Source: CAD feature listing. Evaluate the final solid. Frame: model axes, mm. A direction names the side the tool comes from. Round coordinates to 2 decimals unless told otherwise and drop trailing zeros. Loops run counter-clockwise (first coordinate to the right, second up) from the corner with the lowest first, then second, coordinate; pieces in that order, holes last. Notation, with made-up numbers: (75.25, -38.5) - (99.25, -38.5) arc R8 cw to (99.25, -34.5) - close; hole circle Ø6 at (33, 83.25). An arc over 180 degrees is marked (long way). One line per question, with ' | ' between items.
from build123d import *

# Parameters (mm, degrees)
PAD_DEPTH       = 50
FILLET_R        = 1.5
FILLET001_R     = 1.5
FILLET002_R     = 1.5
FILLET003_R     = 1.5
SKETCH001_R     = 2.1
POCKET_DEPTH    = 50.001
SKETCH002_R     = 2.1
POCKET001_DEPTH = 13.401


with BuildPart() as part:
    # Sketch → Pad (new body)
    with BuildSketch(Plane.XY):
        with BuildLine():
            Line((0, 0), (0, 11.9))
            ThreePointArc((1.5, 13.4), (0.43934, 12.96066), (0, 11.9))
            Line((1.5, 13.4), (48.5, 13.4))
            ThreePointArc((50, 11.9), (49.56066, 12.96066), (48.5, 13.4))
            Line((50, 11.9), (50, 0))
            Line((49, 0), (50, 0))
            Line((49, 11.9), (49, 0))
            ThreePointArc((49, 11.9), (48.853553, 12.253553), (48.5, 12.4))
            Line((1.5, 12.4), (48.5, 12.4))
            ThreePointArc((1.5, 12.4), (1.146447, 12.253553), (1, 11.9))
            Line((1, 0), (1, 11.9))
            Line((0, 0), (1, 0))
        make_face()
    extrude(amount=PAD_DEPTH)

    # Fillet
    fillet_edges = [part.edges().sort_by_distance(p)[0] for p in [
        (49.5, 0, 0),
    ]]
    fillet(fillet_edges, radius=FILLET_R)

    # Fillet001
    fillet001_edges = [part.edges().sort_by_distance(p)[0] for p in [
        (0.5, 0, 0),
    ]]
    fillet(fillet001_edges, radius=FILLET001_R)

    # Fillet002
    fillet002_edges = [part.edges().sort_by_distance(p)[0] for p in [
        (49.5, 0, 50),
    ]]
    fillet(fillet002_edges, radius=FILLET002_R)

    # Fillet003
    fillet003_edges = [part.edges().sort_by_distance(p)[0] for p in [
        (0.5, 0, 50),
    ]]
    fillet(fillet003_edges, radius=FILLET003_R)

    # Sketch001 → Pocket (cut, through all)
    with BuildSketch(Plane(origin=(0, 0, 0), x_dir=(0, -1, 0), z_dir=(-1, 0, 0))):
        with Locations((-5, 5)):
            Circle(SKETCH001_R)
        with Locations((-5, 15)):
            Circle(SKETCH001_R)
        with Locations((-5, 25)):
            Circle(SKETCH001_R)
        with Locations((-5, 35)):
            Circle(SKETCH001_R)
        with Locations((-5, 45)):
            Circle(SKETCH001_R)
    extrude(amount=-POCKET_DEPTH, mode=Mode.SUBTRACT)

    # Sketch002 → Pocket001 (cut, through all)
    with BuildSketch(Plane(origin=(0, 13.4, 0), x_dir=(-1, 0, 0), z_dir=(0, 1, 0))):
        with Locations((-5, 5)):
            Circle(SKETCH002_R)
        with Locations((-5, 15)):
            Circle(SKETCH002_R)
        with Locations((-5, 25)):
            Circle(SKETCH002_R)
        with Locations((-5, 35)):
            Circle(SKETCH002_R)
        with Locations((-5, 45)):
            Circle(SKETCH002_R)
        with Locations((-15, 45)):
            Circle(SKETCH002_R)
        with Locations((-25, 45)):
            Circle(SKETCH002_R)
        with Locations((-35, 45)):
            Circle(SKETCH002_R)
        with Locations((-45, 45)):
            Circle(SKETCH002_R)
        with Locations((-15, 35)):
            Circle(SKETCH002_R)
        with Locations((-25, 35)):
            Circle(SKETCH002_R)
        with Locations((-35, 35)):
            Circle(SKETCH002_R)
        with Locations((-45, 35)):
            Circle(SKETCH002_R)
        with Locations((-15, 25)):
            Circle(SKETCH002_R)
        with Locations((-25, 25)):
            Circle(SKETCH002_R)
        with Locations((-35, 25)):
            Circle(SKETCH002_R)
        with Locations((-45, 25)):
            Circle(SKETCH002_R)
        with Locations((-15, 15)):
            Circle(SKETCH002_R)
        with Locations((-25, 15)):
            Circle(SKETCH002_R)
        with Locations((-35, 15)):
            Circle(SKETCH002_R)
        with Locations((-45, 15)):
            Circle(SKETCH002_R)
        with Locations((-15, 5)):
            Circle(SKETCH002_R)
        with Locations((-25, 5)):
            Circle(SKETCH002_R)
        with Locations((-35, 5)):
            Circle(SKETCH002_R)
        with Locations((-45, 5)):
            Circle(SKETCH002_R)
    extrude(amount=-POCKET001_DEPTH, mode=Mode.SUBTRACT)


solid = part.part
1. Access query for faces 4 (the flat face through (49, 7.4, 24.6)), 5 (the cylindrical face through (22.997, 12.907, 5.631)). Directions: +Z, -Z, +X, -X, +Y, -Y. A direction counts if a zero-diameter tool reaches every point of the face in a straight line with its end or side. Return the directions, or none.
Worked out:
face 4: +Z, -Z, -Y | face 5: +Y, -Y
2. Contact query for a flat-ended pin moving along its axis: P1, Ø5.5, axis at x = 5, z = 15, coming from the -Y side. Output: stop coordinate, or through.
Worked out:
P1: stops at y = 12.4
3. Material intervals for probe 1 along Z at (x, y) = (15, 12.8); probe 2 along X at (y, z) = (7, 9); probe 3 along Y at (x, z) = (31.5, 43.5), sorted ascending.
Worked out:
probe 1: z = 0 to 2.9, 7.1 to 12.9, 17.1 to 22.9, 27.1 to 32.9, 37.1 to 42.9, 47.1 to 50 | probe 2: x = 0 to 1, 49 to 50 | probe 3: y = 12.4 to 13.4
4. Section query A-A, the plane x = 35. Return loops of the section in (y, z), plus the area to 3 significant figures.
Worked out:
outline: (12.4, 0) - (13.4, 0) - (13.4, 2.9) - (12.4, 2.9) - close; (12.4, 7.1) - (13.4, 7.1) - (13.4, 12.9) - (12.4, 12.9) - close; (12.4, 17.1) - (13.4, 17.1) - (13.4, 22.9) - (12.4, 22.9) - close; (12.4, 27.1) - (13.4, 27.1) - (13.4, 32.9) - (12.4, 32.9) - close; (12.4, 37.1) - (13.4, 37.1) - (13.4, 42.9) - (12.4, 42.9) - close; (12.4, 47.1) - (13.4, 47.1) - (13.4, 50) - (12.4, 50) - close | area: 29.0 mm2
5. Section query C-C, the plane z = 29.5. Return loops of the section in (x, y), plus the area to 3 significant figures.
Worked out:
outline: (0, 0) - (1, 0) - (1, 11.9) arc R0.5 cw to (1.5, 12.4) - (48.5, 12.4) arc R0.5 cw to (49, 11.9) - (49, 0) - (50, 0) - (50, 11.9) arc R1.5 ccw to (48.5, 13.4) - (1.5, 13.4) arc R1.5 ccw to (0, 11.9) - close | area: 73.9 mm2
6. Section query B-B, the plane y = 5. Give the number of separate pieces and of enclosed holes in the cut face, plus the area to 3 significant figures.
Worked out:
separate pieces: 12 | enclosed holes: 0 | area: 58.0 mm2
7. Mould query, pull axis Y, two halves, no side actions, for faces 1 (the cylindrical face through (49.49, 3.87, 16.77)), 2 (the cylindrical face through (42.997, 12.907, 15.631)), 3 (the cylindrical face through (49.57, 12.95, 24.65)). Classes: released by +Y, released by -Y, zero draft, split by the parting line, or undercut.
Worked out:
face 1: undercut | face 2: zero draft | face 3: released by +Y
